Input: dimensioned drawing with shaded views. Units: mm. Origin: part minimum x, y, z. A direction names the side the tool comes from. Coordinates: 2 decimals unless noted, no trailing zeros. Loops run counter-clockwise (first coordinate to the right, second up) from the corner with the lowest first, then second, coordinate; pieces in that order, holes last.
Item 1: Ray query, line 1 along Y through (x, z) = (10, 5.25); line 2 along Y through (x, z) = (6, 33). Return the intervals inside material, ascending.
Item 2: Pull-direction query (Y, two-part tool) for the marked faces 1, 2, 3 and 4; classes: released by +Y, released by -Y, zero draft, split by the parting line, or undercut.
Item 3: Section B-B on x = 2.75. Return loops of the section in (y, z).
Item 4: Section A-A on y = 10. Return loops of the section in (x, z).
Item 5: Contact query for flat-ended pins moving along their axis: P1, Ø3, axis at x = 15.5, z = 7, coming from the -Y side; P2, Ø5, axis at x = 8, z = 28, coming from the +Y side; P3, Ø10, axis at y = 11, z = 26.5, coming from the -X side. Output: stop coordinate, or through.
Item 6: Reachability of the marked faces 5, 6, 7, 8 and 9 from +Z, -Z, +X, -X, +Y, -Y: full face, straight path, thin tool, end or side. Return the list, or none.
Item 7: Section D-D on z = 15. Return loops of the section in (x, y).
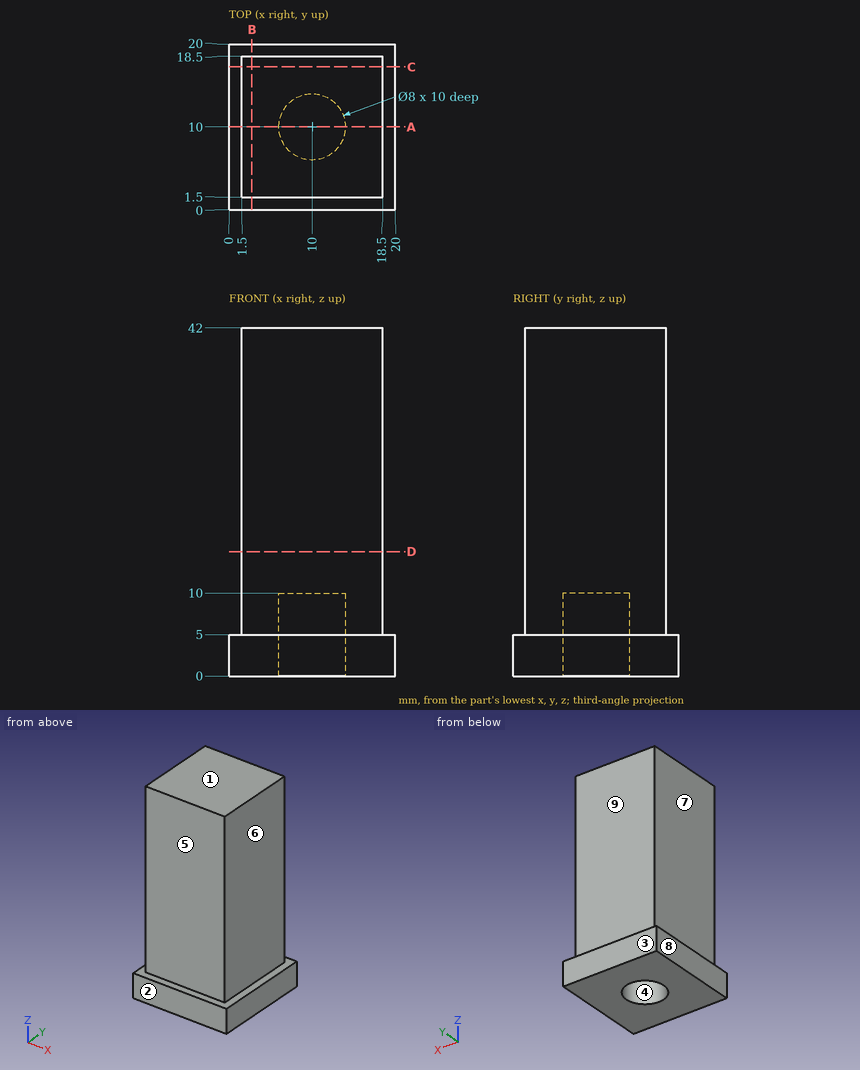
Results found:
1. line 1: y = 1.5 to 6, 14 to 18.5
1. line 2: y = 1.5 to 18.5
2. face 1: zero draft
2. face 2: released by -Y
2. face 3: released by +Y
2. face 4: undercut
3. outline: (0, 0) - (20, 0) - (20, 5) - (18.5, 5) - (18.5, 42) - (1.5, 42) - (1.5, 5) - (0, 5) - close
4. outline: (0, 0) - (6, 0) - (6, 10) - (14, 10) - (14, 0) - (20, 0) - (20, 5) - (18.5, 5) - (18.5, 42) - (1.5, 42) - (1.5, 5) - (0, 5) - close
5. P1: stops at y = 1.5
5. P2: stops at y = 18.5
5. P3: stops at x = 1.5
6. face 5: +Z, +X, -X, -Y
6. face 6: +Z, +X, +Y, -Y
6. face 7: +Z, -X, +Y, -Y
6. face 8: +Z, -Z, -X, +Y, -Y
6. face 9: +Z, +X, -X, +Y
7. outline: (1.5, 1.5) - (18.5, 1.5) - (18.5, 18.5) - (1.5, 18.5) - close
